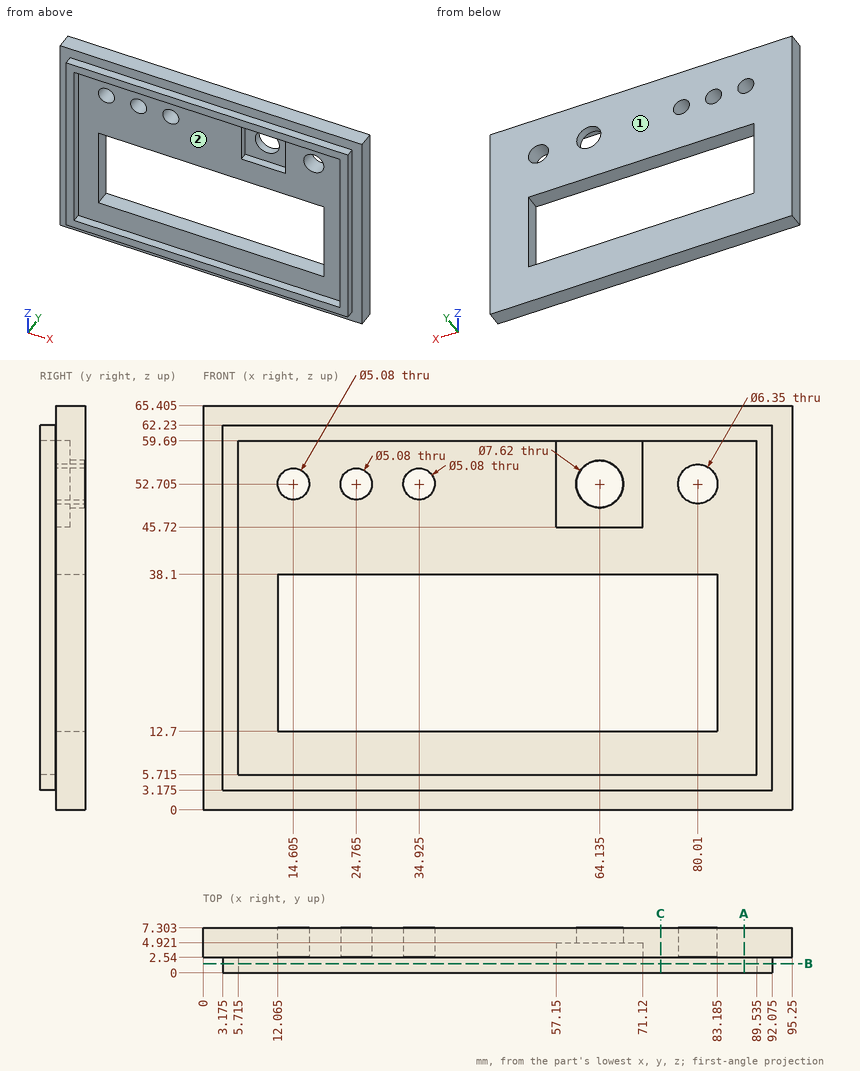
Check sheet for the drawn part. Datum: minimum x, y, z corner. Units: mm. Coordinates: 2 decimals unless noted, no trailing zeros. Order: outer loops, then holes, each group sorted by start corner. A loop starts at its lowest first (then second) coordinate and runs counter-clockwise, first axis right, second up. Notation, with made-up numbers: (21.5, 8.25) -> (27.5, 8.25) arc R18 ccw to (27.5, 42.25) -> close; hole circle Ø6 at (-10.5, -18). An arc over 180 degrees is marked (long way). Write each question's results on one line, items separated by ' | '. Start each with the question number.
1) Draft check along X on the marked faces 1 and 2. Enter one of: pulls with the +X half, pulls with the -X half, needs draft (parallel to the pull), parting line crosses it, or undercut.
2) Depth check by flat-ended pin: pin 1 (1.3 mm diameter, centred on x = 37.5, y = 0.5, fed in from +Z); pin 2 (1 mm diameter, centred on x = 16.5, z = 13, fed in from -Y); pin 3 (3 mm diameter, centred on y = 1, z = 32, fed in from -X) (1 decimal); pin 4 (8 mm diameter, centred on x = 14.605, z = 52.705, fed in from +Y). Enter the tip coordinate at first touch or a pass-through.
3) Section check C-C (x = 74). Enter the section's corners in (y, z) (1 decimal).
4) Section check B-B (y = 1.5). Enter the section's corners in (x, z) (1 decimal).
5) Material ranges on line 1 along Z through (x, y) = (67.5, 4.5) (1 decimal); line 2 along Z through (x, y) = (80.01, 6.15) (1 decimal); line 3 along Z through (x, y) = (72, 6.75) (1 decimal), recorded low to high.
6) Section check A-A (x = 87.5). Enter the section's corners in (y, z) (1 decimal).
Checked values:
1) face 1: needs draft | face 2: undercut
2) pin 1: z = 62.23 | pin 2: y = 2.54 | pin 3: x = 3.2 | pin 4: y = 7.3
3) outline: (0, 3.2) -> (2.5, 3.2) -> (2.5, 0) -> (7.3, 0) -> (7.3, 12.7) -> (2.5, 12.7) -> (2.5, 5.7) -> (0, 5.7) -> close; (0, 59.7) -> (2.5, 59.7) -> (2.5, 38.1) -> (7.3, 38.1) -> (7.3, 65.4) -> (2.5, 65.4) -> (2.5, 62.2) -> (0, 62.2) -> close
4) outline: (3.2, 3.2) -> (92.1, 3.2) -> (92.1, 62.2) -> (3.2, 62.2) -> close; hole (5.7, 5.7) -> (89.5, 5.7) -> (89.5, 59.7) -> (5.7, 59.7) -> close
5) line 1: 0 to 12.7, 38.1 to 45.7, 59.7 to 65.4 | line 2: 0 to 12.7, 38.1 to 49.5, 55.9 to 65.4 | line 3: 0 to 12.7, 38.1 to 65.4
6) outline: (0, 3.2) -> (2.5, 3.2) -> (2.5, 0) -> (7.3, 0) -> (7.3, 65.4) -> (2.5, 65.4) -> (2.5, 62.2) -> (0, 62.2) -> (0, 59.7) -> (2.5, 59.7) -> (2.5, 5.7) -> (0, 5.7) -> close
